Read the model definition and answer for the solid it produces. Units are mm, in the model's axes. Face numbers are marked on the shaded views. A direction names the side the tool comes from. Give positions to 0.01 mm unless a question says otherwise; leave off trailing zeros. Loops run counter-clockwise (first coordinate to the right, second up) from the corner with the lowest first, then second, coordinate; pieces in that order, holes last. Notation, with made-up numbers: (22.5, 65) -> (74.5, 65) arc R19 ccw to (74.5, 89) -> close; hole circle Ø10 at (65.5, 16). An arc over 180 degrees is marked (long way). Write each question's results on one line, items separated by ' | '. Start each with the question number.
Item 1: Section D-D on x = -25 is taken. Write down the section's boundary in (y, z), and give its area (3 significant figures).
Item 2: Find the intervals of material crossed by line 1 (Y direction, x = 1, z = 0); line 2 (Y direction, x = 8, z = 23); line 3 (Y direction, x = 7, z = -21.5), in increasing order.
Item 3: Which of the six approach directions +Z, -Z, +X, -X, +Y, -Y give full straight-line access (tool end or side, diameter ignored) to the marked faces 4 and 5?
Item 4: Determine the mould class of the marked faces 1, 2 and 3 for opening direction Z: +Z half, -Z half, draft (parallel to the pull), parting line (faces both ways), or undercut.
Item 5: Section C-C on x = -6 is taken. Write down the section's boundary in (y, z).
Item 6: Each of these flat-tipped pins is pushed along its axis until it touches: P1, Ø1, axis at x = -20.5, y = 6.5, coming from the +Z side; P2, Ø3, axis at x = -1, z = 6, coming from the -Y side; P3, Ø12, axis at x = -20, y = -6, coming from the -Z side. Where does it stop, or does it pass through?
```python
from build123d import *


with BuildPart() as f1:
    # F0 (on Front) → F1 (revolve)
    with BuildSketch(Plane.XZ):
        with BuildLine():
            ThreePointArc((-30.735126, -14.345073), (-30.183512, -15.724301), (-28.832915, -16.342715))
            Line((-28.832915, -16.342715), (-7.235178, -17.4))
            Line((-7.235178, -17.4), (0.764822, -23.264802))
            Line((0.764822, -23.264802), (0.764822, -33.75))
            Line((0.764822, -33.75), (8.764822, -33.75))
            Line((8.764822, -33.75), (8.764822, -30.75))
            Line((8.764822, -30.75), (4.764822, -29.899774))
            Line((4.764822, -29.899774), (4.764822, -25.6))
            Line((4.764822, -25.6), (8.764822, -25.6))
            Line((8.764822, -25.6), (14.264822, -24.25))
            Line((14.264822, -24.25), (14.264822, -21.5))
            Line((14.264822, -21.5), (8.264822, -20.5))
            Line((8.264822, -20.5), (6, -15))
            Line((6, -15), (0, -15))
            Line((0, -15), (0, 0))
            Line((0, 0), (-30.735126, 0))
            Line((-30.735126, 0), (-30.735126, -14.345073))
        make_face()
    revolve(axis=Axis((-8.246858, 0, 0), (1, 0, 0)))


solid = f1.part
```
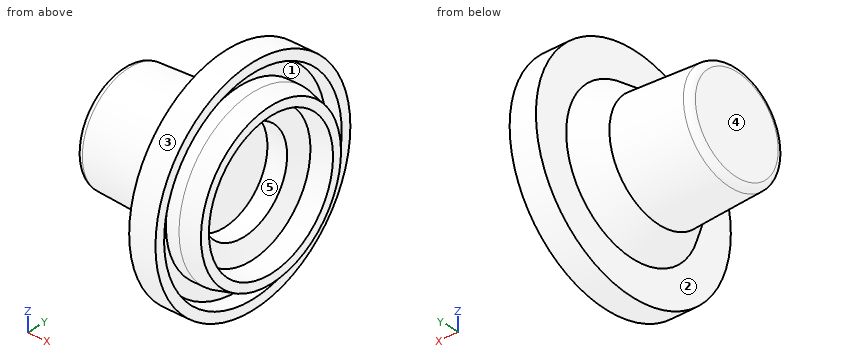
Findings:
1) outline: circle Ø33.06 at (0, 0) | area: 858 mm2
2) line 1: -33.75 to -15, 15 to 33.75 | line 2: -24.7 to -20.16, -11.24 to 11.24, 20.16 to 24.7 | line 3: -26.02 to -21.46, -13.9 to 13.9, 21.46 to 26.02
3) face 4: +Z, -Z, -X, +Y, -Y | face 5: +X
4) face 1: undercut | face 2: draft | face 3: parting line
5) outline: circle Ø36.61 at (0, 0)
6) P1: z = 15.64 | P2: y = -22.34 | P3: z = -16.91
